from build123d import *

# Parameters (mm, degrees)
SKETCH1_W                   = 70
SKETCH1_H                   = 125
BOSS_EXTRUDE1_DEPTH         = 2
LO_XUYEN_M3_D3_4_DEPTH      = 72.660658663
LO_XUYEN_M3_D3_4_DEPTH_BACK = 72.660658663
SKETCH2_R                   = 1.7
THAN_RANH_DEPTH             = 72.660658663
THAN_RANH_DEPTH_BACK        = 72.660658663
SKETCH3_W                   = 5
SKETCH3_H                   = 15
DAU_RANH_R2_5_DEPTH         = 72.660658663
DAU_RANH_R2_5_DEPTH_BACK    = 72.660658663
SKETCH4_R                   = 2.5


with BuildPart() as part:
    # Sketch1 → Boss-Extrude1 (new body)
    with BuildSketch(Plane.XY):
        Rectangle(SKETCH1_W, SKETCH1_H)
    extrude(amount=-BOSS_EXTRUDE1_DEPTH)

    # Sketch2 → Lo_xuyen_M3_D3_4 (cut, two sides: drawn at the far end of the back side and taken through both)
    with BuildSketch(Plane.XY.offset(-LO_XUYEN_M3_D3_4_DEPTH_BACK)):
        with Locations((-30, -55)):
            Circle(SKETCH2_R)
        with Locations((-30, -37.5)):
            Circle(SKETCH2_R)
        with Locations((-30, 37.5)):
            Circle(SKETCH2_R)
        with Locations((-30, 55)):
            Circle(SKETCH2_R)
        with Locations((30, -55)):
            Circle(SKETCH2_R)
        with Locations((30, -37.5)):
            Circle(SKETCH2_R)
        with Locations((30, 37.5)):
            Circle(SKETCH2_R)
        with Locations((30, 55)):
            Circle(SKETCH2_R)
    extrude(amount=LO_XUYEN_M3_D3_4_DEPTH + LO_XUYEN_M3_D3_4_DEPTH_BACK, mode=Mode.SUBTRACT)

    # Sketch3 → Than_ranh (cut, two sides: drawn at the far end of the back side and taken through both)
    with BuildSketch(Plane.XY.offset(-THAN_RANH_DEPTH_BACK)):
        with Locations((-25, -17.5)):
            Rectangle(SKETCH3_W, SKETCH3_H)
        with Locations((-25, 17.5)):
            Rectangle(SKETCH3_W, SKETCH3_H)
        with Locations((25, -17.5)):
            Rectangle(SKETCH3_W, SKETCH3_H)
        with Locations((25, 17.5)):
            Rectangle(SKETCH3_W, SKETCH3_H)
    extrude(amount=THAN_RANH_DEPTH + THAN_RANH_DEPTH_BACK, mode=Mode.SUBTRACT)

    # Sketch4 → Dau_ranh_R2_5 (cut, two sides: drawn at the far end of the back side and taken through both)
    with BuildSketch(Plane.XY.offset(-DAU_RANH_R2_5_DEPTH_BACK)):
        with Locations((-25, -25)):
            Circle(SKETCH4_R)
        with Locations((-25, -10)):
            Circle(SKETCH4_R)
        with Locations((-25, 10)):
            Circle(SKETCH4_R)
        with Locations((-25, 25)):
            Circle(SKETCH4_R)
        with Locations((25, -25)):
            Circle(SKETCH4_R)
        with Locations((25, -10)):
            Circle(SKETCH4_R)
        with Locations((25, 10)):
            Circle(SKETCH4_R)
        with Locations((25, 25)):
            Circle(SKETCH4_R)
    extrude(amount=DAU_RANH_R2_5_DEPTH + DAU_RANH_R2_5_DEPTH_BACK, mode=Mode.SUBTRACT)


solid = part.part
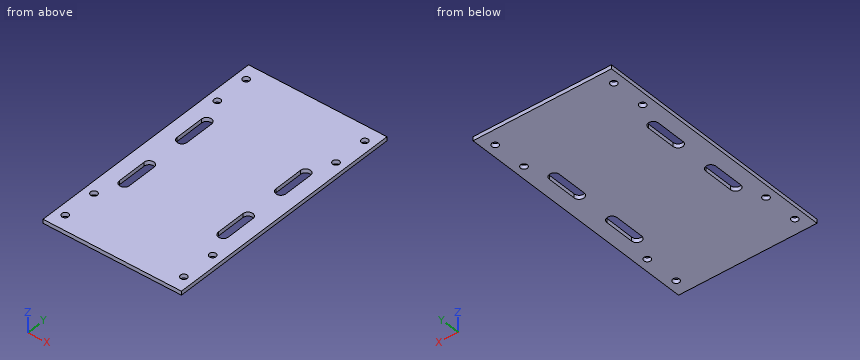
Geometry: final body of the model. Coordinates: model frame, mm. Give positions to 0.01 mm unless a question says otherwise; leave off trailing zeros. Loops run counter-clockwise (first coordinate to the right, second up) from the corner with the lowest first, then second, coordinate; pieces in that order, holes last. Notation, with made-up numbers: (9.5, 10.25) - (67.5, 10.25) arc R28 ccw to (67.5, 34.25) - close; hole circle Ø4 at (22, 15.5). An arc over 180 degrees is marked (long way). Answer as CSV lines item,"result". Start each with the question number.
1. Section C-C, the plane z = -1.55. Give the number of separate pieces and of enclosed holes in the cut face, plus the area to 3 significant figures.
2. Ray query, L1, parallel to Y at x = 30, z = -0.55; L2, parallel to X at y = 18, z = -0.7; L3, parallel to X at y = 37.5, z = -0.55. Return the intervals inside material, ascending.
3. Section A-A, the plane y = 37.5. Return loops of the section in (x, z).
4. Section B-B, the plane x = -25. Return loops of the section in (y, z).
5. Pin query (flat end, axial travel): P1, Ø3, axis at x = 30, y = 55, coming from the +Z side. Return the tip coordinate at first contact, or that it passes through.
Answers:
1,separate pieces,"1"
1,enclosed holes,"12"
1,area,"8,300 mm2"
2,L1,"y = -62.5 to -56.7, -53.3 to -39.2, -35.8 to 35.8, 39.2 to 53.3, 56.7 to 62.5"
2,L2,"x = -35 to -27.5, -22.5 to 22.5, 27.5 to 35"
2,L3,"x = -35 to -31.7, -28.3 to 28.3, 31.7 to 35"
3,outline,"(-35, -2) - (-31.7, -2) - (-31.7, 0) - (-35, 0) - close; (-28.3, -2) - (28.3, -2) - (28.3, 0) - (-28.3, 0) - close; (31.7, -2) - (35, -2) - (35, 0) - (31.7, 0) - close"
4,outline,"(-62.5, -2) - (-27.5, -2) - (-27.5, 0) - (-62.5, 0) - close; (-7.5, -2) - (7.5, -2) - (7.5, 0) - (-7.5, 0) - close; (27.5, -2) - (62.5, -2) - (62.5, 0) - (27.5, 0) - close"
5,P1,"passes through"
